Here's how the part is built. I have some questions about the finished solid (model axes, mm). Round coordinates to 2 decimals unless told otherwise and drop trailing zeros. Order: outer loops, then holes, each group sorted by start corner. A loop starts at its lowest first (then second) coordinate and runs counter-clockwise, first axis right, second up. Notation, with made-up numbers: M 34,37.25 L 53,37.25 A10 ccw 53,52.25 Z; hole C -14,5 d6. An arc over 180 degrees is marked long. Write item = value, one per line. Start each with the question number.
Item 1: I want a section at A-A, the plane z = 0. List the corners of the cut face in (x, y) for me.
Item 2: I want a section at D-D, the plane z = -58. List the corners of the cut face in (x, y) for me.
Item 3: Please list where these lines run through material, in increasing order: L1, parallel to Z at x = 0, y = -2.5; L2, parallel to Y at x = 0.3, z = -94; L3, parallel to Z at x = -1.4, y = 2.
Item 4: I want a section at C-C, the plane x = 0.5. State how many separate pieces and enclosed holes the cut face has, plus the area to 3 significant figures.
Item 5: I want a section at B-B, the plane z = -95.75. List the corners of the cut face in (x, y) for me.
```python
from build123d import *

# Parameters (mm, degrees)
SKETCH1_R                  = 11.1125
SKETCH1_R_2                = 4.7625
BOSS_EXTRUDE1_DEPTH        = 1.5875
M3X0_5_TAPPED_HOLE1_D      = 2.5
M4_CLEARANCE_HOLE1_D       = 4.5
F_8_32_TAPPED_HOLE1_D      = 3.4544
F_1_4_0_2500_DOWEL_HOLE1_D = 6.35
F_1_5MM_START              = -1.5875
F_1_5MM_DOWEL_SLOT1_DEPTH  = 3.175
M4_CLEARANCE_HOLE2_D       = 4.3


# Read off the part's stored shape, not the designer's step: Ø1.5mm Dowel Slot1
with BuildPart() as part:
    # Sketch1 → Boss-Extrude1 (new, symmetric)
    with BuildSketch(Plane(origin=(0, 0, 0), x_dir=(0, 0, -1), z_dir=(1, 0, 0))):
        with BuildLine():
            ThreePointArc((77.61368545, 44.94589464), (75.573628084, 45.000402813), (73.589867092, 44.521343816))
            Line((73.589867092, 44.521343816), (-5.407259882, 13.991481))
            ThreePointArc((-5.407259882, 13.991481), (-14.935591096, -1.388567103), (-2.735294118, -14.748497079))
            Line((-2.735294118, -14.748497079), (79.438235294, -29.988610727))
            ThreePointArc((79.438235294, -29.988610727), (104.085761469, -23.790412126), (115.481107121, -1.073363244))
            ThreePointArc((115.481107121, -1.073363244), (105.257248721, 29.103257737), (77.61368545, 44.94589464))
        make_face()
        Circle(SKETCH1_R, mode=Mode.SUBTRACT)
        with Locations((85, 0)):
            Circle(SKETCH1_R_2, mode=Mode.SUBTRACT)
    extrude(amount=BOSS_EXTRUDE1_DEPTH, both=True)

    # M3x0.5 Tapped Hole1 (through all)
    with Locations(Plane(origin=(1.5875, 0, 0), x_dir=(0, 0, -1), z_dir=(1, 0, 0))):
        with Locations((66.583175665, -4.32590816), (73.896496396, 15.316824335)):
            Hole(M3X0_5_TAPPED_HOLE1_D / 2)

    # M4 Clearance Hole1 (through all)
    with Locations(Plane(origin=(1.5875, 0, 0), x_dir=(0, 0, -1), z_dir=(1, 0, 0))):
        with Locations((95.75, 18.619546181), (95.75, -18.619546181)):
            Hole(M4_CLEARANCE_HOLE1_D / 2)

    # #8-32 Tapped Hole1 (through all)
    with Locations(Plane(origin=(1.5875, 0, 0), x_dir=(0, 0, -1), z_dir=(1, 0, 0))):
        with Locations((76.388124081, 37.280752399)):
            Hole(F_8_32_TAPPED_HOLE1_D / 2)

    # 1/4 (0.2500) Dowel Hole1 (through all)
    with Locations(Plane(origin=(1.5875, 0, 0), x_dir=(0, 0, -1), z_dir=(1, 0, 0))):
        with Locations((59.252323656, 30.844807364)):
            Hole(F_1_4_0_2500_DOWEL_HOLE1_D / 2)

    # Ø1.5mm Dowel Slot1 outline → Ø1.5mm Dowel Slot1 (cut)
    with BuildSketch(Plane.YZ.offset(F_1_5MM_START)):
        with BuildLine():
            Line((-1.15508269, -29.534569304), (-9.512564368, -27.984569304))
            ThreePointArc((-9.512564368, -27.984569304), (-10.386753928, -28.585229452), (-9.78609378, -29.459419012))
            Line((-9.78609378, -29.459419012), (-1.428612102, -31.009419012))
            ThreePointArc((-1.428612102, -31.009419012), (-0.554422542, -30.408758864), (-1.15508269, -29.534569304))
        make_face()
        with BuildLine():
            Line((0.668446721, -19.702237918), (-7.689034957, -18.152237918))
            ThreePointArc((-7.689034957, -18.152237918), (-8.563224517, -18.752898066), (-7.962564368, -19.627087626))
            Line((-7.962564368, -19.627087626), (0.39491731, -21.177087626))
            ThreePointArc((0.39491731, -21.177087626), (1.269106869, -20.576427477), (0.668446721, -19.702237918))
        make_face()
    extrude(amount=F_1_5MM_DOWEL_SLOT1_DEPTH, mode=Mode.SUBTRACT)

    # M4 Clearance Hole2 (through all)
    with Locations(Plane(origin=(1.5875, 0, 0), x_dir=(0, 0, -1), z_dir=(1, 0, 0))):
        with Locations((68.173492099, 32.295918862), (85.614306674, 39.965207417), (83.535698104, 21.026374654)):
            Hole(M4_CLEARANCE_HOLE2_D / 2)


solid = part.part
```
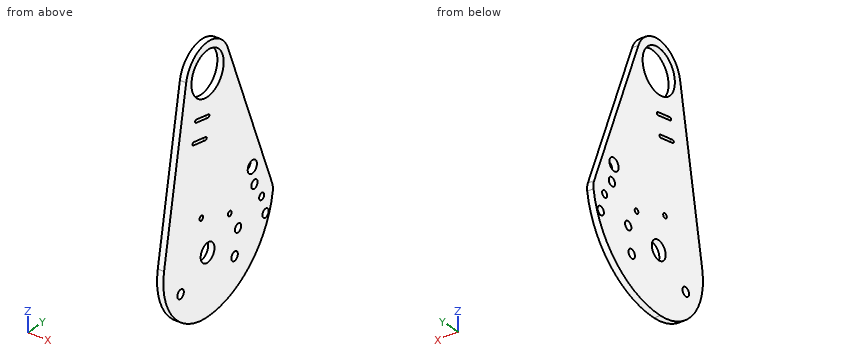
Filled in:
q1.outline = M -1.59,-15.26 L 1.59,-15.26 L 1.59,-11.11 L -1.59,-11.11 Z; M -1.59,11.11 L 1.59,11.11 L 1.59,16.08 L -1.59,16.08 Z
q2.outline = M -1.59,-26.01 L 1.59,-26.01 L 1.59,27.93 L -1.59,27.93 Z; M -1.59,33.76 L 1.59,33.76 L 1.59,38.5 L -1.59,38.5 Z
q3.L1 = -115.4 to -89.05, -80.95 to -30.81, -29.29 to -20.64, -19.11 to -10.83, 10.83 to 14.79
q3.L2 = -29.14 to -20.03, -17.21 to 17.21, 20.03 to 38.89
q3.L3 = -115.48 to -89.32, -80.68 to -10.93, 10.93 to 14.87
q4.separate_pieces = 1
q4.enclosed_holes = 13
q4.area = 6,140 mm^2
q5.outline = M -1.59,-28.54 L 1.59,-28.54 L 1.59,-20.87 L -1.59,-20.87 Z; M -1.59,-16.37 L 1.59,-16.37 L 1.59,16.37 L -1.59,16.37 Z; M -1.59,20.87 L 1.59,20.87 L 1.59,37.76 L -1.59,37.76 Z
